Model file for the job. Use its own axes, mm. Give positions to 0.01 mm unless a question says otherwise; leave off trailing zeros. Loops run counter-clockwise (first coordinate to the right, second up) from the corner with the lowest first, then second, coordinate; pieces in that order, holes last. Notation, with made-up numbers: (38.5, 29.25) - (55.5, 29.25) arc R24 ccw to (55.5, 67.25) - close; hole circle Ø2 at (68, 81.5). An arc over 180 degrees is marked (long way). Answer as CSV lines item,"result". Start each with the question number.
Item 1: Drill centre lines: L1, parallel to Y at x = 14, z = 1.6; L2, parallel to Y at x = 3, z = 0.3; L3, parallel to X at y = 56.5, z = 1.25. Where is each one in solid material? Low to high. Write a range as from..to.
Item 2: Saw through at B-B on y = 45. Give the cut face in (x, z), plus the area to 3 significant figures.
Item 3: Saw through at C-C on z = -0.65. Give the cut face in (x, y).
Item 4: Saw through at A-A on x = -12. Give the cut face in (y, z).
Item 5: Pull direction X, two halves, no side cores. Call faces 1 (the flat face through (-0.3, 56.1, 0)), 2 (the flat face through (-23, 63, -2)), 3 (the flat face through (-24.5, 30, 1)): pulls with the +X half, pulls with the -X half, needs draft (parallel to the pull), parting line crosses it, or undercut.
Item 6: Saw through at D-D on x = 32. Give the cut face in (y, z), plus the area to 3 significant figures.
Item 7: Pin check, flat tip, straight feed: pin 1 (1.5 mm diameter, centred on y = 46, z = -0.5, fed in from +X). Stop position of the tip, or through.
from build123d import *

# Parameters (mm, degrees)
F0_W     = 120
F0_H     = 70
F1_DEPTH = 2
F3_DEPTH = 1
F4_W     = 4
F4_H     = 4
F5_DEPTH = 2


with BuildPart() as f1:
    # F0 (on Top) → F1 (new body)
    with BuildSketch(Plane.XY):
        with Locations((35.5, 30)):
            Rectangle(F0_W, F0_H)
        Polygon((2, 49), (2, 58), (85, 58), (85, 2), (-14, 2), (-14, 49), align=None, mode=Mode.SUBTRACT)
    extrude(amount=F1_DEPTH)

    # F2 (on face) → F3 (cut)
    with BuildSketch(Plane(origin=(0, 0, 0), x_dir=(1, 0, 0), z_dir=(0, 0, -1))):
        Polygon((95.5, 0), (-16, 0), (-16, -51), (0, -51), (0, -60), (95.5, -60), align=None)
    extrude(amount=-F3_DEPTH, mode=Mode.SUBTRACT)

    # F4 (on face) → F5 (join)
    with BuildSketch(Plane(origin=(0, 0, 0), x_dir=(1, 0, 0), z_dir=(0, 0, -1))):
        with Locations((-22.5, 3)):
            Rectangle(F4_W, F4_H)
        with Locations((-22.5, -63)):
            Rectangle(F4_W, F4_H)
        with Locations((93.5, 3)):
            Rectangle(F4_W, F4_H)
        with Locations((93.5, -63)):
            Rectangle(F4_W, F4_H)
    extrude(amount=F5_DEPTH)


solid = f1.part
Responses:
1,L1,"-5..2, 58..65"
1,L2,"-5..0, 60..65"
1,L3,"-24.5..2, 85..95.5"
2,outline,"(-24.5, 0) - (-16, 0) - (-16, 1) - (-14, 1) - (-14, 2) - (-24.5, 2) - close; (85, 1) - (95.5, 1) - (95.5, 2) - (85, 2) - close"
2,area,"29.5 mm2"
3,outline,"(-24.5, -5) - (-20.5, -5) - (-20.5, -1) - (-24.5, -1) - close; (-24.5, 61) - (-20.5, 61) - (-20.5, 65) - (-24.5, 65) - close; (91.5, -5) - (95.5, -5) - (95.5, -1) - (91.5, -1) - close; (91.5, 61) - (95.5, 61) - (95.5, 65) - (91.5, 65) - close"
4,outline,"(-5, 0) - (0, 0) - (0, 1) - (2, 1) - (2, 2) - (-5, 2) - close; (49, 1) - (51, 1) - (51, 0) - (65, 0) - (65, 2) - (49, 2) - close"
5,face 1,"undercut"
5,face 2,"needs draft"
5,face 3,"pulls with the -X half"
6,outline,"(-5, 0) - (0, 0) - (0, 1) - (2, 1) - (2, 2) - (-5, 2) - close; (58, 1) - (60, 1) - (60, 0) - (65, 0) - (65, 2) - (58, 2) - close"
6,area,"24.0 mm2"
7,pin 1,"x = -16"
